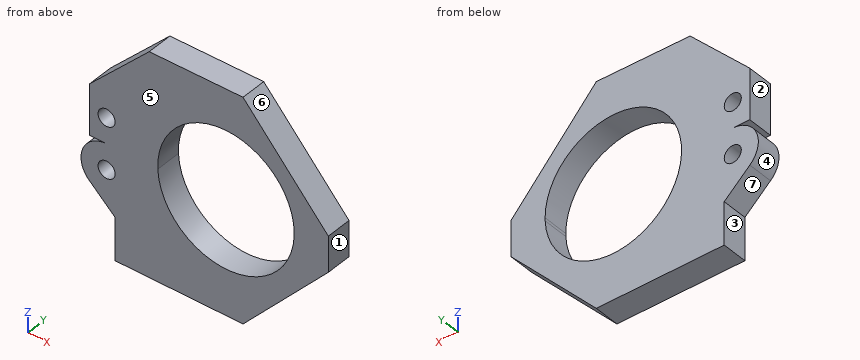
```python
from build123d import *

# Parameters (mm, degrees)
F0_R     = 3.175
F1_DEPTH = 9.525
F2_DEPTH = 9.525


with BuildPart() as f1:
    # F0 (on Front) → F1 (new body)
    with BuildSketch(Plane.XZ):
        with BuildLine():
            Line((-23.813147, 35.108108), (-46.038147, 12.51385))
            Line((-46.038147, 12.51385), (-46.038147, -6.35))
            Line((-46.038147, -6.35), (-39.688147, -6.35))
            Line((-39.688147, -6.35), (-20.612767, -6.35))
            ThreePointArc((-20.612767, -6.35), (4.194114, 20.178848), (30.161853, -5.214807))
            ThreePointArc((30.161853, -5.214807), (30.155507, -5.782545), (30.136473, -6.35))
            Line((30.136473, -6.35), (42.861853, -6.35))
            Line((42.861853, -6.35), (42.861853, 0))
            Line((42.861853, 0), (11.111853, 35.395849))
            Line((11.111853, 35.395849), (-23.813147, 35.108108))
        make_face()
        with Locations((-39.688147, 3.175)):
            Circle(F0_R, mode=Mode.SUBTRACT)
    extrude(amount=F1_DEPTH)

    # F0 (on Front) → F2 (join)
    with BuildSketch(Plane.XZ):
        with BuildLine():
            Line((-20.612767, -6.35), (-39.688147, -6.35))
            ThreePointArc((-39.688147, -6.35), (-48.586139, -12.47627), (-46.038147, -22.974516))
            Line((-46.038147, -22.974516), (-36.513147, -31.75))
            Line((-36.513147, -31.75), (-36.513147, -47.625))
            Line((-36.513147, -47.625), (11.111853, -47.625))
            Line((11.111853, -47.625), (42.861853, -13.260503))
            Line((42.861853, -13.260503), (42.861853, -6.35))
            Line((42.861853, -6.35), (30.136473, -6.35))
            ThreePointArc((30.136473, -6.35), (4.761853, -30.614807), (-20.612767, -6.35))
        make_face()
        with Locations((-39.688147, -15.875)):
            Circle(F0_R, mode=Mode.SUBTRACT)
    extrude(amount=F2_DEPTH)


solid = f1.part
```
CAD build for the part. Positions are in the model's coordinates, mm. Face numbers are marked on the shaded views. A direction names the side the tool comes from. Round coordinates to 2 decimals unless told otherwise and drop trailing zeros. Loops run counter-clockwise (first coordinate to the right, second up) from the corner with the lowest first, then second, coordinate; pieces in that order, holes last. Notation, with made-up numbers: M 16,26.25 L 50,26.25 A18 cw 50,45.25 Z; hole C -6.5,74.25 d7. An arc over 180 degrees is marked long. Return JSON: item names as keys, results as strings. Group by question number.
(1) Saw through at B-B, the plane z = 18.5. List the corners of the cut face in (x, y) (3 decimals).
(2) Wall check: probe 1 along X at (y, z) = (-1, -16); probe 2 along X at (y, z) = (-1.25, -15); probe 3 along Z at (x, y) = (-39, -8.75). Give the ranges that are in metal, low to high. Write a range as [from, to].
(3) Drop flat-ended pins along their axis: P1, Ø4, axis at y = -2, z = -25, coming from the -X side; P2, Ø1.9, axis at x = -44, y = -6.5, coming from the -Z side; P3, Ø3, axis at y = -5, z = -43, coming from the -X side. Give the stop position or say it passes through.
(4) Mould opens along Z. For the marked faces 4, 5, 6 and 7 say: +Z half, -Z half, draft (parallel to the pull), parting line (faces both ways), or undercut.
(5) Tool access for the marked faces 1, 2 and 3: list every direction of +Z, -Z, +X, -X, +Y, -Y with a clear straight run to the whole face (end or side of a thin tool).
(6) Saw through at D-D, the plane x = -41.5. List the corners of the cut face in (y, z) (3 decimals).
(7) Saw through at C-C, the plane y = -2.75. Give the number of separate pieces and of enclosed holes in the cut face, and give its area (3 significant figures).
(8) Saw through at A-A, the plane x = -7.5. List the corners of the cut face in (y, z) (1 decimal), and give its area (3 significant figures).
Answer list:
{
 "1": {"outline": "M -40.15,-9.525 L -4.336,-9.525 L -4.336,0 L -40.15,0 Z; M 13.86,-9.525 L 26.267,-9.525 L 26.267,0 L 13.86,0 Z"},
 "2": {"probe 1": "[-49.21, -42.86], [-36.52, -18.23], [27.76, 40.33]", "probe 2": "[-49.17, -42.74], [-36.64, -18.68], [28.2, 41.25]", "probe 3": "[-29.46, -18.97], [-12.78, 0.08], [6.27, 19.67]"},
 "3": {"P1": "x = -46.01", "P2": "z = -25.73", "P3": "x = -36.51"},
 "4": {"face 4": "undercut", "face 5": "draft", "face 6": "+Z half", "face 7": "-Z half"},
 "5": {"face 1": "+Z, -Z, +X, +Y, -Y", "face 2": "+Z, -X, +Y, -Y", "face 3": "-Z, -X, +Y, -Y"},
 "6": {"outline": "M -9.525,-27.156 L 0,-27.156 L 0,-18.482 L -9.525,-18.482 Z; M -9.525,-13.268 L 0,-13.268 L 0,-6.524 L -9.525,-6.524 Z; M -9.525,-6.35 L 0,-6.35 L 0,0.568 L -9.525,0.568 Z; M -9.525,5.782 L 0,5.782 L 0,17.127 L -9.525,17.127 Z"},
 "7": {"separate pieces": "1", "enclosed holes": "3", "area": "3,750 mm2"},
 "8": {"outline": "M -9.5,-47.6 L 0,-47.6 L 0,-27.5 L -9.5,-27.5 Z; M -9.5,17 L 0,17 L 0,35.2 L -9.5,35.2 Z", "area": "366 mm2"}
}
